Check sheet for the drawn part. Datum: minimum x, y, z corner. Units: mm. A direction names the side the tool comes from. Coordinates: 2 decimals unless noted, no trailing zeros. Loops run counter-clockwise (first coordinate to the right, second up) from the corner with the lowest first, then second, coordinate; pieces in that order, holes last.
Q1. Mould release check, pull along Y, two halves, no side actions. Record for the marked faces 1, 2, 3 and 4: +Y half, -Y half, draft (parallel to the pull), parting line (faces both ways), or undercut.
Q2. Material ranges on probe 1 along X at (y, z) = (11.5, 4) (1 decimal); probe 2 along X at (y, z) = (16.5, 3); probe 3 along Y at (x, z) = (23, 3.75), recorded low to high.
Q3. Access from +Z, -Z, +X, -X, +Y, -Y to the whole of each face (thin tool, end or side, straight path). Record for the marked faces 5 and 6.
Q4. Go/stop test with flat-tipped pins: P1, Ø12, axis at x = 33.5, y = 7.5, coming from the +Z side; P2, Ø4.5, axis at x = 6, y = 11.75, coming from the +Z side. Record where each tip stops, or that it passes through.
Q5. Sectioned sample at A-A (x = 46.5). Enter the section's corners in (y, z).
Q6. Sectioned sample at C-C (z = 1). Enter the section's corners in (x, y), then the cut area to 3 significant figures.
Q7. Sectioned sample at D-D (z = 5). Enter the section's corners in (x, y), then the cut area to 3 significant figures.
Q8. Sectioned sample at B-B (y = 11.75). Enter the section's corners in (x, z).
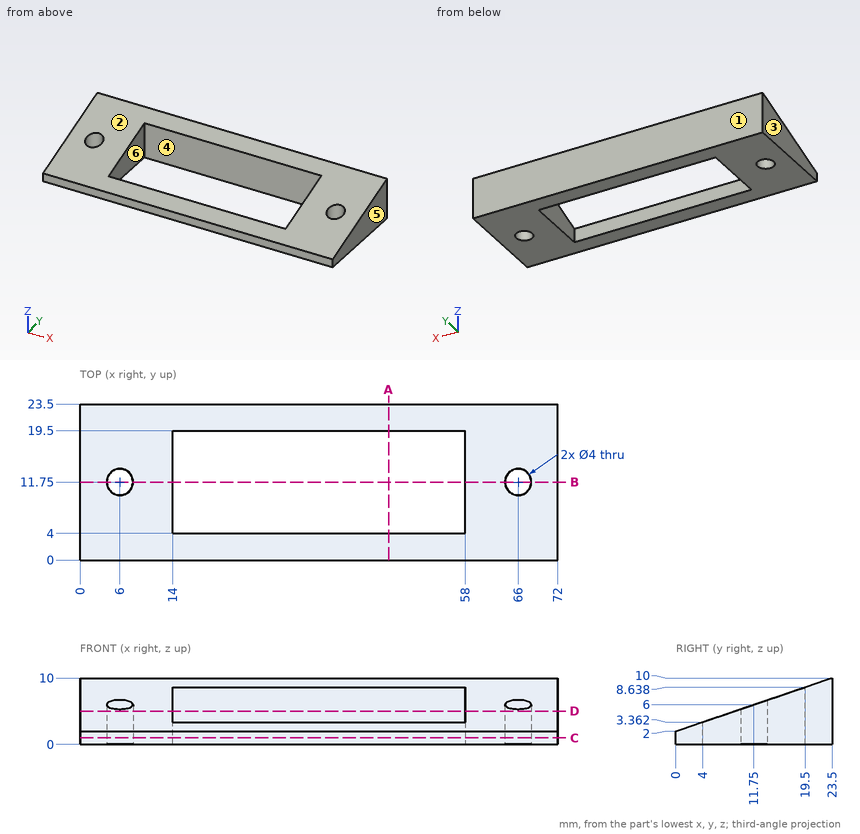
Geometry check:
1. face 1: +Y half
1. face 2: -Y half
1. face 3: draft
1. face 4: undercut
2. probe 1: x = 0 to 4, 8 to 14, 58 to 64, 68 to 72
2. probe 2: x = 0 to 14, 58 to 72
2. probe 3: y = 19.5 to 23.5
3. face 5: +Z, -Z, +X, +Y, -Y
3. face 6: +Z, -Z
4. P1: stops at z = 3.36
4. P2: stops at z = 6.77
5. outline: (0, 0) - (4, 0) - (4, 3.36) - (0, 2) - close; (19.5, 0) - (23.5, 0) - (23.5, 10) - (19.5, 8.64) - close
6. outline: (0, 0) - (72, 0) - (72, 23.5) - (0, 23.5) - close; hole circle Ø4 at (6, 11.75); hole (14, 4) - (58, 4) - (58, 19.5) - (14, 19.5) - close; hole circle Ø4 at (66, 11.75)
6. area: 985 mm2
7. outline: (0, 8.81) - (14, 8.81) - (14, 19.5) - (58, 19.5) - (58, 8.81) - (72, 8.81) - (72, 23.5) - (0, 23.5) - close; hole circle Ø4 at (6, 11.75); hole circle Ø4 at (66, 11.75)
7. area: 562 mm2
8. outline: (0, 0) - (4, 0) - (4, 6) - (0, 6) - close; (8, 0) - (14, 0) - (14, 6) - (8, 6) - close; (58, 0) - (64, 0) - (64, 6) - (58, 6) - close; (68, 0) - (72, 0) - (72, 6) - (68, 6) - close
